The listing builds one solid part. Answer for the finished solid, in the listing's coordinates (mm). A direction names the side the tool comes from. Round coordinates to 2 decimals unless told otherwise and drop trailing zeros. Write each loop counter-clockwise with the first axis right and the second up, starting at its lowest first coordinate (ties: lowest second). Pieces come first, ordered by that corner, then holes. Notation, with made-up numbers: M 82.25,73.5 L 138.25,73.5 A33 ccw 138.25,104.5 Z; hole C 34,-37 d5. An arc over 180 degrees is marked long. Answer as CSV lines item,"result". Start each with the question number.
Autodesk Inventor part; units mm, degrees
ref_plane "YZ Plane" through (0, 0, 0) normal (1, 0, 0) x (0, 1, 0)
ref_plane "XZ Plane" through (0, 0, 0) normal (0, 1, 0) x (-1, 0, 0)
ref_plane "XY Plane" through (0, 0, 0) normal (0, 0, 1) x (1, 0, 0)
sketch "Sketch1" plane through (0, 0, 0) normal (0, 1, 0) x (-1, 0, 0)
  line L0 (58, 27) -> (-58, 27)
  line L1 (-58, 27) -> (-58, -27)
  line L2 (-58, -27) -> (58, -27)
  line L3 (58, -27) -> (58, 27)
  line L4 (58, 27) -> (-58, -27) construction
  line L5 (-58, 27) -> (58, -27) construction
  point P0 (0, 0)
  dimension "d0" = 116
  dimension "d1" = 54
extrude "Body" add sketch "Sketch1" along normal mid plane 10
sketch "Sketch12" plane through (0, 5, 0) normal (0, 1, 0) x (1, 0, 0)
  line L0 (58, 27) -> (-58, 27)
  circle A0 centre (-50.8, 25.4) radius 6
  line L1 (-58, -27) -> (-58, 27)
  line L2 (-58, 0) -> (58, 0)
  line L3 (58, 27) -> (58, -27)
  line L4 (-58, -27) -> (58, -27)
  line L5 (0, -27) -> (0, 27)
  circle A1 centre (50.8, 25.4) radius 6
  circle A2 centre (-50.8, -25.4) radius 6
  circle A3 centre (50.8, -25.4) radius 6
  line L6 (-50.8, 25.4) -> (50.8, 25.4)
  line L7 (-50.8, -25.4) -> (50.8, -25.4)
  circle A4 centre (0, 25.4) radius 6
  circle A5 centre (0, -25.4) radius 6
  point P0 (0, 0)
  dimension "d40" = 25.4
  dimension "d49" = 50.8
  dimension "d57" = 12
extrude "Screw clamp boss" add sketch "Sketch12" against normal up to surface (10 mm away) contours A1 L0 | L0 A1 | A4 L6 L5 L0 | L0 A4 | A5 L7 L5 | L5 L7 A5 | A4 L6 L5 | L5 L6 A4 | A3 L4 | L4 A3 | L5 L6 A4 L0 | L7 A5 L4 L5 | L5 L4 A5 L7 | A0 L0 | L0 A0 | A2 L4 | L4 A2 | L4 A5
sketch "Sketch15" plane through (0, 5, 0) normal (0, 1, 0) x (1, 0, 0)
  circle A0 centre (0, 25.4) radius 2.55
  arc A1 (5.7827, 27) -> (-5.7827, 27) centre (0, 25.4) ccw
  circle A2 centre (-50.8, 25.4) radius 2.55
  arc A3 (-45.0173, 27) -> (-56.5827, 27) centre (-50.8, 25.4) ccw
  line L0 (55.75, -18.75) -> (-55.75, -18.75)
  line L1 (0, -18.75) -> (0, 18.75)
  line L2 (-55.75, 18.75) -> (55.75, 18.75)
  line L3 (-58, 27) -> (-58, -27)
  line L4 (-58, 0) -> (58, 0)
  line L5 (58, -27) -> (58, 27)
  circle A4 centre (50.8, 25.4) radius 2.55
  circle A5 centre (0, -25.4) radius 2.55
  circle A6 centre (-50.8, -25.4) radius 2.55
  circle A7 centre (50.8, -25.4) radius 2.55
  point P0 (0, 0)
  dimension "d60" = 5.1
extrude "Screw Clamp Hole" cut sketch "Sketch15" against normal through all
sketch "Sketch17" plane through (0, 5, 0) normal (0, 1, 0) x (1, 0, 0)
  line L0 (-46.5, -5.5) -> (46.5, -5.5)
  line L1 (46.5, -5.5) -> (46.5, 5.5)
  line L2 (46.5, 5.5) -> (-46.5, 5.5)
  line L3 (-46.5, 5.5) -> (-46.5, -5.5)
  line L4 (-46.5, -5.5) -> (46.5, 5.5) construction
  line L5 (46.5, -5.5) -> (-46.5, 5.5) construction
  line L6 (-38, -5.5) -> (-26, -5.5)
  line L7 (-26, -5.5) -> (-26, 5.5)
  line L8 (-26, 5.5) -> (-38, 5.5)
  line L9 (-38, 5.5) -> (-38, -5.5)
  arc A0 (-5.7827, -27) -> (5.7827, -27) centre (0, -25.4) ccw
  circle A1 centre (0, 25.4) radius 2.55
  line L10 (0, -25.4) -> (0, 25.4)
  line L11 (26, -5.5) -> (38, -5.5)
  line L12 (38, -5.5) -> (38, 5.5)
  line L13 (38, 5.5) -> (26, 5.5)
  line L14 (26, 5.5) -> (26, -5.5)
  point P0 (0, 0)
  dimension "d70" = 93
  dimension "d71" = 11
  dimension "d72" = 38
  dimension "d73" = 12
extrude "Main Window" cut sketch "Sketch17" against normal through all contours L7 L2 L10 L0 | L10 L2 L14 L0
sketch "Sketch18" plane through (0, 5, 0) normal (0, 1, 0) x (1, 0, 0)
  line L0 (-46.5, -5.5) -> (46.5, -5.5)
  line L1 (46.5, -5.5) -> (46.5, 5.5)
  line L2 (46.5, 5.5) -> (-46.5, 5.5)
  line L3 (-46.5, 5.5) -> (-46.5, -5.5)
  line L4 (-46.5, -5.5) -> (46.5, 5.5) construction
  line L5 (46.5, -5.5) -> (-46.5, 5.5) construction
  line L6 (-38, -5.5) -> (-26, -5.5)
  line L7 (-26, -5.5) -> (-26, 5.5)
  line L8 (-26, 5.5) -> (-38, 5.5)
  line L9 (-38, 5.5) -> (-38, -5.5)
  arc A0 (-5.7827, -27) -> (5.7827, -27) centre (0, -25.4) ccw
  circle A1 centre (0, 25.4) radius 2.55
  line L10 (0, -25.4) -> (0, 25.4)
  line L11 (26, -5.5) -> (38, -5.5)
  line L12 (38, -5.5) -> (38, 5.5)
  line L13 (38, 5.5) -> (26, 5.5)
  line L14 (26, 5.5) -> (26, -5.5)
  point P0 (0, 0)
  point P1 (0, 0)
  dimension "d76" = 93
  dimension "d77" = 11
  dimension "d78" = 38
  dimension "d79" = 12
extrude "Inelt Outlet Access" cut sketch "Sketch18" against normal through all contours L3 L2 L9 L0 | L12 L2 L1 L0
properties part number "Top Clamp 6_6"
Q1. Find section C-C (x = -21). Determine the outline of the cut face in (y, z).
Q2. Find section B-B (z = -25.4). Determine the outline of the cut face in (x, y), plus the area to 3 significant figures.
Q3. For faces 4 (the face through (-25, 0, -27)), 5 (the face through (-42, 0, 5.5)), 6 (the face through (1, 5, 7)), 7 (the face through (25, 0, 27)), determine the directions among +Z, -Z, +X, -X, +Y, -Y from which every point of the face is accessible in a straight line to the end or side of a thin tool.
Q4. The mould has two halves that part along X. Classify faces 1 (the face through (58, 0, 0)), 2 (the face through (1, -5, 7)), 3 (the face through (26, 0, -27)): +X half, -X half, draft (parallel to the pull), parting line (faces both ways), or undercut.
Q5. Find section D-D (y = -2). Count the separate pieces of the cut face and the enclosed holes in it, plus the area to 3 significant figures.
Q6. Each of these flat-tipped pins is pushed along its axis until it touches: P1, Ø3, axis at x = -13, y = 0, coming from the -Z side; P2, Ø6.5, axis at x = 50.8, z = -25.4, coming from the +Y side; P3, Ø4, axis at x = 43.5, y = -1.5, coming from the +Z side. Where does it stop, or does it pass through?
Q7. Find section A-A (x = 50.8). Determine the outline of the cut face in (y, z).
Q8. Straight lines are drawn through the part: L1, parallel to Z at x = -50.8, y = 0.25; L2, parallel to X at y = -0.5, z = -25.4; L3, parallel to Z at x = 0, y = -2. For each, find the intervals that lie inside material, in ascending order.
Reported:
1,outline,"M -5,-27 L 5,-27 L 5,-5.5 L -5,-5.5 Z; M -5,5.5 L 5,5.5 L 5,27 L -5,27 Z"
2,outline,"M -58,-5 L -53.35,-5 L -53.35,5 L -58,5 Z; M -48.25,-5 L -2.55,-5 L -2.55,5 L -48.25,5 Z; M 2.55,-5 L 48.25,-5 L 48.25,5 L 2.55,5 Z; M 53.35,-5 L 58,-5 L 58,5 L 53.35,5 Z"
2,area,"1,010 mm2"
3,face 4,"-Z, +Y, -Y"
3,face 5,"+Y, -Y"
3,face 6,"+Z, -Z, +X, -X, +Y"
3,face 7,"+Z, +Y, -Y"
4,face 1,"+X half"
4,face 2,"draft"
4,face 3,"undercut"
5,separate pieces,"1"
5,enclosed holes,"9"
5,area,"5,610 mm2"
6,P1,"stops at z = -27"
6,P2,"stops at y = 5"
6,P3,"stops at z = 28.21"
7,outline,"M -5,-31.4 L 5,-31.4 L 5,-27.95 L -5,-27.95 Z; M -5,-22.85 L 5,-22.85 L 5,22.85 L -5,22.85 Z; M -5,27.95 L 5,27.95 L 5,31.4 L -5,31.4 Z"
8,L1,"z = -31.4 to -27.95, -22.85 to 22.85, 27.95 to 31.4"
8,L2,"x = -58 to -53.35, -48.25 to -2.55, 2.55 to 48.25, 53.35 to 58"
8,L3,"z = -31.4 to -27.95, -22.85 to -5.5, 5.5 to 22.85, 27.95 to 31.4"
